Verification items for the finished model (mm, model axes). Face numbers are marked on the shaded views. Coordinates: 2 decimals unless noted, no trailing zeros. Write each loop counter-clockwise with the first axis right and the second up, starting at its lowest first coordinate (ties: lowest second). Pieces come first, ordered by that corner, then holes. Notation, with made-up numbers: (24, 60) -> (33, 60) arc R13 cw to (33, 80) -> close; hole circle Ø5 at (-35.75, 89.25). An arc over 180 degrees is marked (long way). Answer in a Markdown table with one row per item.
```python
from build123d import *

# Parameters (mm, degrees)
SKETCH1_R                       = 17.78
SKETCH1_R_2                     = 15.875
BOSS_EXTRUDE1_DEPTH             = 22.225
CHAMFER4_SIZE                   = 1.905
CHAMFER4_SIZE2                  = 1.099852263
F_27_0_144_DIAMETER_HOLE1_D     = 3.6576
F_27_0_144_DIAMETER_HOLE1_DEPTH = 25.4
F_27_0_144_DIAMETER_HOLE1_TIP   = 1.0988539


with BuildPart() as part:
    # Sketch1 → Boss-Extrude1 (new body)
    with BuildSketch(Plane.XY):
        Circle(SKETCH1_R)
        Circle(SKETCH1_R_2, mode=Mode.SUBTRACT)
    extrude(amount=BOSS_EXTRUDE1_DEPTH)

    # Chamfer4
    chamfer4_edges = [part.edges().sort_by_distance(p)[0] for p in [
        (-17.78, 0, 22.225),
    ]]
    chamfer4_side = [part.faces().sort_by_distance(p)[0] for p in [
        (-17.78, 0, 11.1125),
    ]]
    chamfer(chamfer4_edges, length=CHAMFER4_SIZE, length2=CHAMFER4_SIZE2, reference=chamfer4_side[0])

    # #27 (0.144) Diameter Hole1
    with Locations(Plane(origin=(0, 17.78, 4.445), x_dir=(1, 0, 0), z_dir=(0, 1, 0))):
        with Locations((0, 0)):
            Hole(F_27_0_144_DIAMETER_HOLE1_D / 2, depth=F_27_0_144_DIAMETER_HOLE1_DEPTH)
            with Locations((0, 0, -(F_27_0_144_DIAMETER_HOLE1_DEPTH + F_27_0_144_DIAMETER_HOLE1_TIP / 2))):  # 118° drill point
                Cone(0, F_27_0_144_DIAMETER_HOLE1_D / 2, F_27_0_144_DIAMETER_HOLE1_TIP, mode=Mode.SUBTRACT)


solid = part.part
```
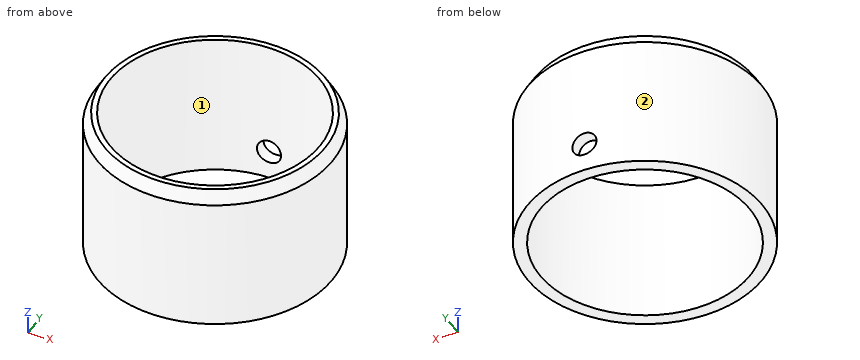
1. Go/stop test with flat-tipped pins: pin 1 (12 mm diameter, centred on x = 11, y = 4, fed in from +Z) (3 decimals); pin 2 (6 mm diameter, centred on x = 9.5, z = 12, fed in from +Y); pin 3 (1.5 mm diameter, centred on x = 12.5, z = 15.5, fed in from -Y); pin 4 (4 mm diameter, centred on y = 14, z = 4, fed in from +X). Record where each tip stops, or that it passes through.
Findings below:
| item | result |
|---|---|
| pin 1 | stops at z = 22.225 |
| pin 2 | stops at y = 16.55 |
| pin 3 | stops at y = -13.34 |
| pin 4 | stops at x = 13.12 |
2. Sectioned sample at C-C, the plane z = 15.75. Record the cut outline in (x, y) (3 decimals), and give its area (3 significant figures).
Findings below:
| item | result |
|---|---|
| outline | circle Ø35.56 at (0, 0); hole circle Ø31.75 at (0, 0) |
| area | 201 mm² |
3. Release check for a two-part mould opening along Y. For the marked faces 1 and 2 record: released by +Y, released by -Y, zero draft, split by the parting line, or undercut.
Findings below:
| item | result |
|---|---|
| face 1 | undercut |
| face 2 | split by the parting line |
4. Material ranges on probe 1 along Y at (x, z) = (0, 9) (3 decimals); probe 2 along Y at (x, z) = (4, 9); probe 3 along X at (y, z) = (5.5, 4.25), recorded low to high. Write a range as from..to.
Findings below:
| item | result |
|---|---|
| probe 1 | y = -17.78..-15.875, 15.875..17.78 |
| probe 2 | y = -17.32..-15.36, 15.36..17.32 |
| probe 3 | x = -16.91..-14.89, 14.89..16.91 |
5. Sectioned sample at B-B, the plane y = 0. Record the cut outline in (x, z) (3 decimals), and give its area (3 significant figures).
Findings below:
| item | result |
|---|---|
| outline | (-17.78, 0) -> (-15.875, 0) -> (-15.875, 22.225) -> (-16.68, 22.225) -> (-17.78, 20.32) -> close; (15.875, 0) -> (17.78, 0) -> (17.78, 20.32) -> (16.68, 22.225) -> (15.875, 22.225) -> close |
| area | 82.6 mm² |
6. Sectioned sample at D-D, the plane z = 5. Record the cut outline in (x, y) (3 decimals).
Findings below:
| item | result |
|---|---|
| outline | (-1.743, 15.779) -> (-1.743, 17.694) arc R17.78 ccw (long way) to (1.743, 17.694) -> (1.743, 15.779) arc R15.875 cw (long way) to start |
7. Sectioned sample at A-A, the plane x = 0. Record the cut outline in (y, z) (3 decimals).
Findings below:
| item | result |
|---|---|
| outline | (-17.78, 0) -> (-15.875, 0) -> (-15.875, 22.225) -> (-16.68, 22.225) -> (-17.78, 20.32) -> close; (15.875, 0) -> (17.78, 0) -> (17.78, 2.616) -> (15.875, 2.616) -> close; (15.875, 6.274) -> (17.78, 6.274) -> (17.78, 20.32) -> (16.68, 22.225) -> (15.875, 22.225) -> close |
